Source: three-view drawing plus pictorial views. Frame: mm from the lowest corner of the part. A direction names the side the tool comes from. Give positions to 0.01 mm unless a question says otherwise; leave off trailing zeros. Loops run counter-clockwise (first coordinate to the right, second up) from the corner with the lowest first, then second, coordinate; pieces in that order, holes last.
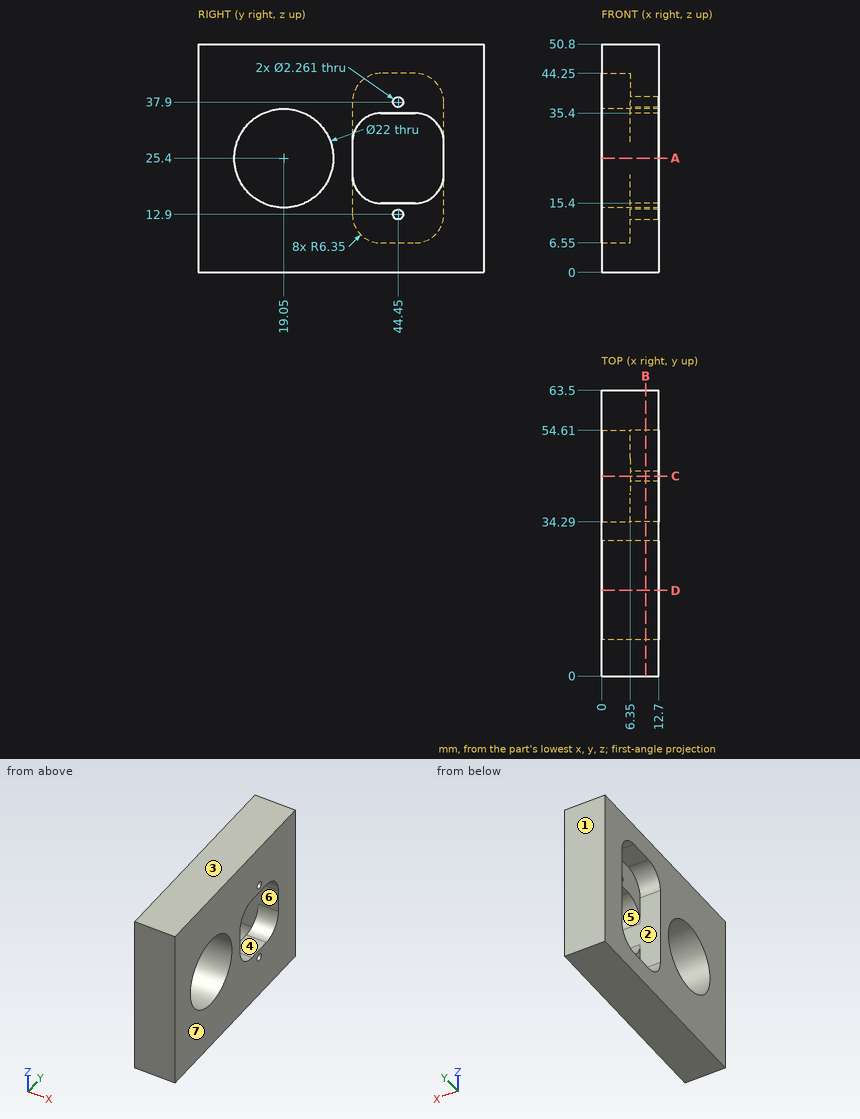
Q1. Section query B-B, the plane x = 9.75. Return loops of the section in (y, z), and give its area (3 significant figures).
Q2. Pin query (flat end, axial travel): pin 1 Ø7.5 at (y, z) = (39.5, 17) entering from -X. Return the tip coordinate at first contact, or that it passes through.
Q3. Section query A-A, the plane z = 25.4. Return loops of the section in (x, y).
Q4. Mould query, pull axis Y, two halves, no side actions, for the marked faces 1, 2, 3 and 4. Classes: +Y half, -Y half, draft (parallel to the pull), parting line (faces both ways), or undercut.
Q5. Section query D-D, the plane y = 19.05. Return loops of the section in (x, z).
Q6. Material intervals for probe 1 along Y at (x, z) = (3.25, 25.4); probe 2 along Y at (x, z) = (2.5, 36.5); probe 3 along Z at (x, y) = (6.75, 41), sorted ascending.
Q7. Reachability of the marked faces 5, 6 and 7 from +Z, -Z, +X, -X, +Y, -Y: full face, straight path, thin tool, end or side. Return the list, or none.
Q8. Section query C-C, the plane y = 44.45. Return loops of the section in (x, z).
Resolved:
1. outline: (0, 0) - (63.5, 0) - (63.5, 50.8) - (0, 50.8) - close; hole circle Ø22 at (19.05, 25.4); hole (34.29, 21.75) arc R6.35 ccw to (40.64, 15.4) - (48.26, 15.4) arc R6.35 ccw to (54.61, 21.75) - (54.61, 29.05) arc R6.35 ccw to (48.26, 35.4) - (40.64, 35.4) arc R6.35 ccw to (34.29, 29.05) - close; hole circle Ø2.26 at (44.45, 12.9); hole circle Ø2.26 at (44.45, 37.9)
1. area: 2,470 mm2
2. pin 1: stops at x = 6.35
3. outline: (0, 0) - (12.7, 0) - (12.7, 8.05) - (0, 8.05) - close; (0, 30.05) - (12.7, 30.05) - (12.7, 34.29) - (0, 34.29) - close; (0, 54.61) - (12.7, 54.61) - (12.7, 63.5) - (0, 63.5) - close
4. face 1: +Y half
4. face 2: undercut
4. face 3: draft
4. face 4: undercut
5. outline: (0, 0) - (12.7, 0) - (12.7, 14.4) - (0, 14.4) - close; (0, 36.4) - (12.7, 36.4) - (12.7, 50.8) - (0, 50.8) - close
6. probe 1: y = 0 to 8.05, 30.05 to 34.29, 54.61 to 63.5
6. probe 2: y = 0 to 34.29, 54.61 to 63.5
6. probe 3: z = 0 to 15.4, 35.4 to 50.8
7. face 5: +X, -X
7. face 6: -X
7. face 7: +Z, -Z, +X, +Y, -Y
8. outline: (0, 0) - (12.7, 0) - (12.7, 11.77) - (6.35, 11.77) - (6.35, 6.55) - (0, 6.55) - close; (0, 44.25) - (6.35, 44.25) - (6.35, 39.03) - (12.7, 39.03) - (12.7, 50.8) - (0, 50.8) - close; (6.35, 14.03) - (12.7, 14.03) - (12.7, 15.4) - (6.35, 15.4) - close; (6.35, 35.4) - (12.7, 35.4) - (12.7, 36.77) - (6.35, 36.77) - close
